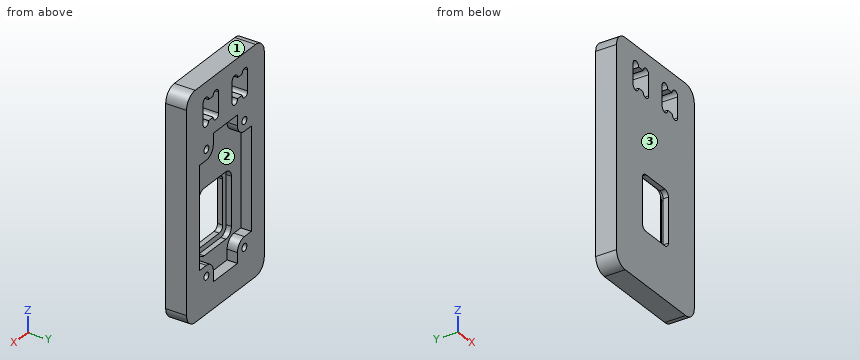
from build123d import *

# Parameters (mm, degrees)
BOSS_EXTRUDE1_DEPTH = 8
CUT_EXTRUDE1_START  = -4
SKETCH3_R           = 1.4
CUT_EXTRUDE1_DEPTH  = 4
CUT_EXTRUDE2_DEPTH  = 2


with BuildPart() as part:
    # Sketch1 → Boss-Extrude1 (new body)
    with BuildSketch(Plane(origin=(0, 0, 0), x_dir=(1, 0, 0), z_dir=(0, 1, 0))):
        with BuildLine():
            Line((25, 41), (-10, 41))
            ThreePointArc((-10, 41), (-13.535533906, 39.535533906), (-15, 36))
            Line((-15, 36), (-15, -40))
            ThreePointArc((-15, -40), (-13.535533906, -43.535533906), (-10, -45))
            Line((-10, -45), (25, -45))
            ThreePointArc((25, -45), (28.535533906, -43.535533906), (30, -40))
            Line((30, -40), (30, 36))
            ThreePointArc((30, 36), (28.535533906, 39.535533906), (25, 41))
        make_face()
        with BuildLine():
            Line((-5.4, -37.8), (-5.4, -30))
            ThreePointArc((-5.4, -30), (-3.8, -28.4), (-2.2, -30))
            Line((-2.2, -30), (0.4, -30))
            ThreePointArc((0.4, -30), (2, -28.4), (3.6, -30))
            Line((3.6, -30), (3.6, -37.8))
            ThreePointArc((3.6, -37.8), (2, -39.4), (0.4, -37.8))
            Line((0.4, -37.8), (-2.2, -37.8))
            ThreePointArc((-2.2, -37.8), (-3.8, -39.4), (-5.4, -37.8))
        make_face(mode=Mode.SUBTRACT)
        with BuildLine():
            Line((11.4, -37.8), (11.4, -30))
            ThreePointArc((11.4, -30), (13, -28.4), (14.6, -30))
            Line((14.6, -30), (17.2, -30))
            ThreePointArc((17.2, -30), (18.8, -28.4), (20.4, -30))
            Line((20.4, -30), (20.4, -37.8))
            ThreePointArc((20.4, -37.8), (18.8, -39.4), (17.2, -37.8))
            Line((17.2, -37.8), (14.6, -37.8))
            ThreePointArc((14.6, -37.8), (13, -39.4), (11.4, -37.8))
        make_face(mode=Mode.SUBTRACT)
        with BuildLine():
            Line((13, 0), (2, 0))
            ThreePointArc((2, 0), (0.585786438, 0.585786438), (0, 2))
            Line((0, 2), (0, 19))
            ThreePointArc((0, 19), (0.585786438, 20.414213562), (2, 21))
            Line((2, 21), (13, 21))
            ThreePointArc((13, 21), (14.414213562, 20.414213562), (15, 19))
            Line((15, 19), (15, 2))
            ThreePointArc((15, 2), (14.414213562, 0.585786438), (13, 0))
        make_face(mode=Mode.SUBTRACT)
    extrude(amount=BOSS_EXTRUDE1_DEPTH)

    # Sketch3 → Cut-Extrude1 (cut)
    # profile 1 of 5: a face of its own
    with BuildSketch(Plane(origin=(0, 8, 0), x_dir=(1, 0, 0), z_dir=(0, 1, 0)).offset(CUT_EXTRUDE1_START)):
        with BuildLine():
            Line((14.5, 31), (0.5, 31))
            Line((0.5, 31), (0.5, 27))
            ThreePointArc((0.5, 27), (-0.671572875, 24.171572875), (-3.5, 23))
            Line((-3.5, 23), (-7.5, 23))
            Line((-7.5, 23), (-7.5, -16))
            Line((-7.5, -16), (-3.5, -16))
            ThreePointArc((-3.5, -16), (-0.671572875, -17.171572875), (0.5, -20))
            Line((0.5, -20), (0.5, -24))
            Line((0.5, -24), (14.5, -24))
            Line((14.5, -24), (14.5, -20))
            ThreePointArc((14.5, -20), (15.671572875, -17.171572875), (18.5, -16))
            Line((18.5, -16), (22.5, -16))
            Line((22.5, -16), (22.5, 23))
            Line((22.5, 23), (18.5, 23))
            ThreePointArc((18.5, 23), (15.671572875, 24.171572875), (14.5, 27))
            Line((14.5, 27), (14.5, 31))
        make_face()
        with BuildLine():
            ThreePointArc((13, 21), (14.414213562, 20.414213562), (15, 19))
            Line((15, 19), (15, 2))
            ThreePointArc((15, 2), (14.414213562, 0.585786438), (13, 0))
            Line((13, 0), (2, 0))
            ThreePointArc((2, 0), (0.585786438, 0.585786438), (0, 2))
            Line((0, 2), (0, 19))
            ThreePointArc((0, 19), (0.585786438, 20.414213562), (2, 21))
            Line((2, 21), (13, 21))
        make_face(mode=Mode.SUBTRACT)
    # profile 2 of 5: a face of its own
    with BuildSketch(Plane(origin=(0, 8, 0), x_dir=(1, 0, 0), z_dir=(0, 1, 0)).offset(CUT_EXTRUDE1_START)):
        with Locations(Location((-3.5, 27, 0), (0, 0, 270))):
            Circle(SKETCH3_R)
    # profile 3 of 5: a face of its own
    with BuildSketch(Plane(origin=(0, 8, 0), x_dir=(1, 0, 0), z_dir=(0, 1, 0)).offset(CUT_EXTRUDE1_START)):
        with Locations(Location((18.5, 27, 0), (0, 0, 270))):
            Circle(SKETCH3_R)
    # profile 4 of 5: a face of its own
    with BuildSketch(Plane(origin=(0, 8, 0), x_dir=(1, 0, 0), z_dir=(0, 1, 0)).offset(CUT_EXTRUDE1_START)):
        with Locations(Location((-3.5, -20, 0), (0, 0, 270))):
            Circle(SKETCH3_R)
    # profile 5 of 5: a face of its own
    with BuildSketch(Plane(origin=(0, 8, 0), x_dir=(1, 0, 0), z_dir=(0, 1, 0)).offset(CUT_EXTRUDE1_START)):
        with Locations(Location((18.5, -20, 0), (0, 0, 270))):
            Circle(SKETCH3_R)
    extrude(amount=CUT_EXTRUDE1_DEPTH, mode=Mode.SUBTRACT)

    # Sketch5 → Cut-Extrude2 (cut)
    with BuildSketch(Plane(origin=(0, 4, 0), x_dir=(1, 0, 0), z_dir=(0, 1, 0))):
        with BuildLine():
            Line((1.2, -2), (13.8, -2))
            ThreePointArc((13.8, -2), (16.0627417, -1.0627417), (17, 1.2))
            Line((17, 1.2), (17, 19.8))
            ThreePointArc((17, 19.8), (16.0627417, 22.0627417), (13.8, 23))
            Line((13.8, 23), (1.2, 23))
            ThreePointArc((1.2, 23), (-1.0627417, 22.0627417), (-2, 19.8))
            Line((-2, 19.8), (-2, 1.2))
            ThreePointArc((-2, 1.2), (-1.0627417, -1.0627417), (1.2, -2))
        make_face()
    extrude(amount=-CUT_EXTRUDE2_DEPTH, mode=Mode.SUBTRACT)


solid = part.part
Input: part model. Units: mm. Frame: model coordinates. Face numbers are marked on the shaded views. Give positions to 0.01 mm unless a question says otherwise; leave off trailing zeros. Order: outer loops, then holes, each group sorted by start corner. A loop starts at its lowest first (then second) coordinate and runs counter-clockwise, first axis right, second up.
Q1. Draft query along Z for the marked faces 1, 2 and 3. Return one class per face: +Z half, -Z half, draft (parallel to the pull), parting line (faces both ways), or undercut.
Checked values:
face 1: +Z half
face 2: undercut
face 3: draft
Q2. Ray query, probe 1 along X at (y, z) = (6.3, -27); probe 2 along X at (y, z) = (7.5, 34); probe 3 along Z at (x, y) = (-4, 1). Return the intervals inside material, ascending.
Checked values:
probe 1: x = -15 to -4.9, -2.1 to 0.5, 14.5 to 17.1, 19.9 to 30
probe 2: x = -15 to -5.4, 3.6 to 11.4, 20.4 to 30
probe 3: z = -41 to 28.41, 39.39 to 45
Q3. Contact query for a flat-ended pin moving along its axis: pin 1 Ø1.7 at (x, z) = (18.5, 20) entering from +Y. Output: stop coordinate, or through.
Checked values:
pin 1: stops at y = 4
Q4. Section B-B on z = -30. Output: boundary loops of the cut face in (x, y).
Checked values:
outline: (-15, 0) - (30, 0) - (30, 8) - (14.5, 8) - (14.5, 4) - (0.5, 4) - (0.5, 8) - (-15, 8) - close
Q5. Section A-A on z = 36.5. Output: boundary loops of the cut face in (x, y), and give its area (3 significant figures).
Checked values:
outline: (-15, 0) - (-5.4, 0) - (-5.4, 8) - (-15, 8) - close; (3.6, 0) - (11.4, 0) - (11.4, 8) - (3.6, 8) - close; (20.4, 0) - (30, 0) - (30, 8) - (20.4, 8) - close
area: 216 mm2
